Here's how the part is built. I have some questions about the finished solid (model axes, mm). A direction names the side the tool comes from. Coordinates: 2 decimals unless noted, no trailing zeros. Write each loop counter-clockwise with the first axis right and the second up, starting at its lowest first coordinate (ties: lowest second). Pieces come first, ordered by that corner, then holes.
from build123d import *

# Parameters (mm, degrees)
F0_W     = 50.882496
F0_H     = 26.710287
F1_DEPTH = 38.1
F3_DEPTH = 12.7


with BuildPart() as f1:
    # F0 (on Front) → F1 (new body)
    with BuildSketch(Plane.XZ):
        with Locations((25.441248, 13.355143)):
            Rectangle(F0_W, F0_H)
    extrude(amount=-F1_DEPTH)

    # F2 (on face) → F3 (cut)
    with BuildSketch(Plane.XY.offset(26.710287)):
        Polygon((31.75, 38.1), (6.35, 0), (38.182496, 0), (50.882496, 19.05), (50.882496, 38.1), align=None)
    extrude(amount=-F3_DEPTH, mode=Mode.SUBTRACT)


solid = f1.part
1. On a 3-axis mill with a long thin cutter (end or side, diameter ignored), from which of +Z, -Z, +X, -X, +Y, -Y can I reach the whole of each face in a straight line? I mean faces 1 (the face through (44.444, 9.392, 20.449)), 2 (the face through (12, 23, 26.71)), 3 (the face through (19.23, 19.32, 20.45)). Say none if no direction works.
2. I want a section at B-B (y = 28.5). List the corners of the cut face in (x, z) for me, then the cut area to 3 significant figures.
3. I want a section at A-A (z = 21). List the corners of the cut face in (x, y) for me, then the cut area to 3 significant figures.
4. If I drill on line 1 (Z direction, x = 35.5, y = 7); line 2 (X direction, y = 17.5, z = 14.25); line 3 (X direction, y = 18.5, z = 18), over which ranges is the centre line in solid material (lowest first)?
5. Thinking about a two-plate mould opening in X: for faces 4 (the face through (25, 0, 11)), 5 (the face through (33, 19, 14.01)), 6 (the face through (0, 19, 13)), which applies, pulls with the +X half, pulls with the -X half, needs draft (parallel to the pull), parting line crosses it, or undercut?
6. For pin 1 Ø1 at (x, z) = (41.5, 15) entering from -Y, with a flat end and sliding along its axis, tell me the tip position at first contact or that it passes through.
7. I want a section at C-C (x = 10.5). List the corners of the cut face in (y, z) for me (3 decimals).
8. I want a section at D-D (y = 16). List the corners of the cut face in (x, z) for me.
Response values:
1. face 1: +Z, +Y
1. face 2: +Z, +X, -X, +Y, -Y
1. face 3: +Z, -Y
2. outline: (0, 0) - (50.88, 0) - (50.88, 14.01) - (25.35, 14.01) - (25.35, 26.71) - (0, 26.71) - close
2. area: 1,030 mm2
3. outline: (0, 0) - (6.35, 0) - (31.75, 38.1) - (0, 38.1) - close; (38.18, 0) - (50.88, 0) - (50.88, 19.05) - close
3. area: 847 mm2
4. line 1: z = 0 to 14.01
4. line 2: x = 0 to 18.02, 49.85 to 50.88
4. line 3: x = 0 to 18.68, 50.52 to 50.88
5. face 4: needs draft
5. face 5: undercut
5. face 6: pulls with the -X half
6. pin 1: stops at y = 0
7. outline: (0, 0) - (38.1, 0) - (38.1, 26.71) - (6.225, 26.71) - (6.225, 14.01) - (0, 14.01) - close
8. outline: (0, 0) - (50.88, 0) - (50.88, 26.71) - (48.85, 26.71) - (48.85, 14.01) - (17.02, 14.01) - (17.02, 26.71) - (0, 26.71) - close
